Part model, mm, in its own coordinate system. Face numbers are marked on the shaded views. A direction names the side the tool comes from. Give positions to 0.01 mm unless a question says otherwise; leave off trailing zeros. Write each loop counter-clockwise with the first axis right and the second up, starting at its lowest first coordinate (ties: lowest second). Pieces come first, ordered by that corner, then holes. Notation, with made-up numbers: (54.25, -34) - (63.25, -34) arc R24 ccw to (63.25, -3) - close; hole circle Ø10 at (7, 5.25). An arc over 180 degrees is marked (long way). Answer as a JSON object with one key per item and string values. Group by question number.
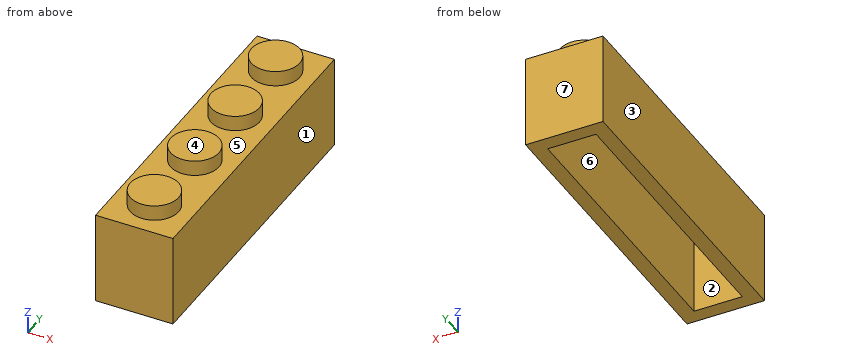
Autodesk Inventor part; units mm, degrees
ref_plane "YZ Plane" through (0, 0, 0) normal (1, 0, 0) x (0, 1, 0)
ref_plane "XZ Plane" through (0, 0, 0) normal (0, 1, 0) x (-1, 0, 0)
ref_plane "XY Plane" through (0, 0, 0) normal (0, 0, 1) x (1, 0, 0)
sketch "Sketch1" plane through (0, 0, 0) normal (0, 0, 1) x (1, 0, 0)
  line L0 (-4, 16) -> (4, 16)
  line L1 (4, 16) -> (4, -16)
  line L2 (4, -16) -> (-4, -16)
  line L3 (-4, -16) -> (-4, 16)
  point P0 (0, 0)
  dimension "d0" = 8
  dimension "d1" = 32
  dimension "d2" = 4
  dimension "d3" = 16
extrude "Extrusion1" add sketch "Sketch1" along normal blind 9.6
shell "Shell1" thickness 1.5 removed faces 1 at (-1.3333, 5.3333, 0)
sketch "Sketch2" plane through (0, 0, 9.6) normal (0, 0, 1) x (1, 0, 0)
  circle A0 centre (0, -12) radius 2.5
  line L0 (4, 16) -> (4, -16)
  line L1 (4, -16) -> (-4, -16)
  dimension "d7" = 5
  dimension "d10" = 4
  dimension "d11" = 4
extrude "Extrusion2" add sketch "Sketch2" along normal blind 1.6
sketch "Sketch3" plane through (2.5, -14.5, 8.1) normal (0, 0, -1) x (-1, 0, 0)
  circle A0 centre (2.5, 2.5) radius 2.5
  circle A1 centre (2.5, 2.5) radius 1.2
  point P0 (2.5, 14.5)
  dimension "d18" = 2.4
extrude "Extrusion3" cut sketch "Sketch3" against normal blind 1.6 contours A1
pattern_linear "Rectangular Pattern1" count 4 spacing 8 along (0, 1, 0) of "Extrusion2", "Extrusion3"
sketch "Sketch4" plane through (2.5, -14.5, 8.1) normal (0, 0, -1) x (-1, 0, 0)
  circle A0 centre (2.5, 10.5) radius 1.2
  circle A1 centre (2.5, 2.5) radius 1.2
  line L0 (0, 29) -> (0, 0)
  line L1 (0, 0) -> (5, 0)
  circle A2 centre (6.5, 6.5) radius 3.15
  circle A3 centre (6.5, 6.5) radius 2.5
  point P0 (2.5, 14.5)
  dimension "d21" = 6.5
  dimension "d22" = 6.5
  dimension "d23" = 10.5
  dimension "d24" = 2.5
  dimension "d25" = 5
  dimension "d26" = 6.3
extrude "Extrusion4" [suppressed]
pattern_linear "Rectangular Pattern2" [suppressed]
equation "\"d0\" = 0.8 * WIDTH"
equation "\"d1\" = 0.8 * LENGTH"
equation "\"d4\" = HEIGHT"
equation "\"d21\" = 0.5 * d23 + 0.5 * d24"
equation "\"d22\" = d21"
equation "\"WIDTH\" = 1"
equation "\"HEIGHT\" = 9.6"
properties part number "3010" material "Steel"
1) Band-saw the part on B-B (y = 7). List the corners of the cut face in (x, z), plus the area to 3 significant figures.
2) Probe line 1 (Y direction, x = 0, z = 8.65); line 2 (X direction, y = 10, z = 1.75); line 3 (Y direction, x = -1.5, z = 7.5). List the from-to ranges inside material, lowest first.
3) Band-saw the part on A-A (z = 2.25). List the corners of the cut face in (x, y), plus the area to 3 significant figures.
4) Which spindle directions (+Z, -Z, +X, -X, +Y, -Y) get a long thin tool onto all of the face, cutting with end or side? Do the marked faces 5, 6 and 7. Say none if no direction does.
5) Mould opens along X. For the marked faces 1, 2, 3 and 4 say: pulls with the +X half, pulls with the -X half, needs draft (parallel to the pull), parting line crosses it, or undercut.
6) Band-saw the part on D-D (y = -12). List the corners of the cut face in (x, z), plus the area to 3 significant figures.
7) Drop flat-ended pins along their axis: P1, Ø1.9, axis at x = 0, y = 4, coming from the -Z side; P2, Ø2, axis at x = -0.5, y = 12.5, coming from the -Z side. Give the stop position or say it passes through.
8) Band-saw the part on C-C (x = 3). List the corners of the cut face in (y, z), plus the area to 3 significant figures.
Verdict:
{
 "1": {"outline": "(-4, 0) - (-2.5, 0) - (-2.5, 8.1) - (2.5, 8.1) - (2.5, 0) - (4, 0) - (4, 9.6) - (-4, 9.6) - close", "area": "36.3 mm2"},
 "2": {"line 1": "-16 to -13.2, -10.8 to -5.2, -2.8 to 2.8, 5.2 to 10.8, 13.2 to 16", "line 2": "-4 to -2.5, 2.5 to 4", "line 3": "-16 to -14.5, 14.5 to 16"},
 "3": {"outline": "(-4, -16) - (4, -16) - (4, 16) - (-4, 16) - close; hole (-2.5, -14.5) - (2.5, -14.5) - (2.5, 14.5) - (-2.5, 14.5) - close", "area": "111 mm2"},
 "4": {"face 5": "+Z", "face 6": "-Z", "face 7": "+Z, -Z, +X, -X, +Y"},
 "5": {"face 1": "pulls with the +X half", "face 2": "undercut", "face 3": "pulls with the -X half", "face 4": "needs draft"},
 "6": {"outline": "(-4, 0) - (-2.5, 0) - (-2.5, 8.1) - (-1.2, 8.1) - (-1.2, 9.7) - (1.2, 9.7) - (1.2, 8.1) - (2.5, 8.1) - (2.5, 0) - (4, 0) - (4, 9.6) - (2.5, 9.6) - (2.5, 11.2) - (-2.5, 11.2) - (-2.5, 9.6) - (-4, 9.6) - close", "area": "40.5 mm2"},
 "7": {"P1": "z = 9.7", "P2": "z = 8.1"},
 "8": {"outline": "(-16, 0) - (16, 0) - (16, 9.6) - (-16, 9.6) - close", "area": "307 mm2"}
}
